Answer from the drawing. Dimensions are ordinates in mm from the lowest x, y and z of the part. A direction names the side the tool comes from. Round coordinates to 2 decimals unless told otherwise and drop trailing zeros. Write each loop counter-clockwise with the first axis right and the second up, starting at its lowest first coordinate (ties: lowest second). Pieces come first, ordered by that corner, then holes. Notation, with made-up numbers: (12, 61) -> (59, 61) arc R26 cw to (59, 75) -> close; hole circle Ø4 at (-14, -28). An arc over 180 degrees is marked (long way). Return JSON: item names as keys, results as strings. Group by question number.
(1) A cutting plane is placed at C-C on z = 441.5. Give the vertices of the cut face in (x, y), then the cut area to 3 significant figures.
(2) Straight lines are drawn through the part: line 1 (Z direction, x = 84, y = 431.5); line 2 (Y direction, x = 386.5, z = 394); line 3 (X direction, y = 801, z = 392). For each, find the intervals that lie inside material, in ascending order.
(3) The mould has two halves that part along Z. Classify the marked faces 3 and 4: released by +Z, released by -Z, zero draft, split by the parting line, or undercut.
(4) A cutting plane is placed at A-A on y = 391.5. Give the vertices of the cut face in (x, z), then the cut area to 3 significant figures.
(5) A cutting plane is placed at D-D on y = 646. Give the vertices of the cut face in (x, z), then the cut area to 3 significant figures.
(6) For the marked faces 1 and 2, determine the directions among +Z, -Z, +X, -X, +Y, -Y from which every point of the face is accessible in a straight line to the end or side of a thin tool.
(7) A cutting plane is placed at B-B on x = 486. Give the vertices of the cut face in (y, z).
(8) Given pin 1 (10 mm diameter, centred on y = 753, z = 78.5, fed in from -X); pin 2 (21 mm diameter, centred on y = 274, z = 9, fed in from +X); pin 3 (12 mm diameter, centred on x = 269, z = 115.5, fed in from +Y), each flat-ended and moving along its own axis, determine where each tip first touches the part or whether it passes through.
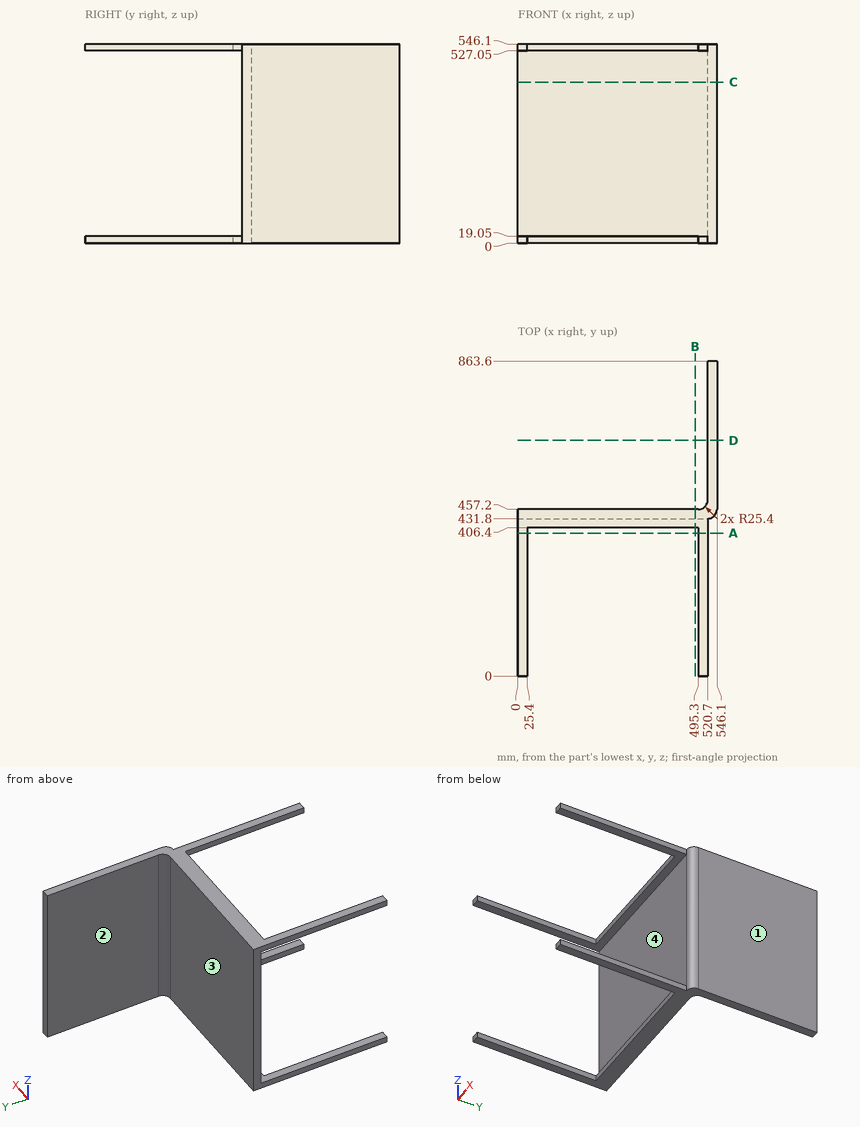
Checks:
{
 "1": {"outline": "(0, 431.8) -> (520.7, 431.8) arc R25.4 ccw to (546.1, 457.2) -> (546.1, 863.6) -> (520.7, 863.6) -> (520.7, 482.6) arc R25.4 cw to (495.3, 457.2) -> (0, 457.2) -> close", "area": "24,200 mm^2"},
 "2": {"line 1": "z = 0 to 19.05, 527.05 to 546.1", "line 2": "y = 431.8 to 457.2", "line 3": "x = 520.7 to 546.1"},
 "3": {"face 3": "zero draft", "face 4": "undercut"},
 "4": {"outline": "(0, 0) -> (25.4, 0) -> (25.4, 19.05) -> (0, 19.05) -> close; (0, 527.05) -> (25.4, 527.05) -> (25.4, 546.1) -> (0, 546.1) -> close; (495.3, 0) -> (520.7, 0) -> (520.7, 19.05) -> (495.3, 19.05) -> close; (495.3, 527.05) -> (520.7, 527.05) -> (520.7, 546.1) -> (495.3, 546.1) -> close", "area": "1,940 mm^2"},
 "5": {"outline": "(520.7, 0) -> (546.1, 0) -> (546.1, 546.1) -> (520.7, 546.1) -> close", "area": "13,900 mm^2"},
 "6": {"face 1": "+Z, -Z, +X, +Y, -Y", "face 2": "+Z, -Z, -X, +Y"},
 "7": {"outline": "(406.4, 0) -> (457.2, 0) -> (457.2, 546.1) -> (406.4, 546.1) -> (406.4, 527.05) -> (431.8, 527.05) -> (431.8, 19.05) -> (406.4, 19.05) -> close"},
 "8": {"pin 1": "stops at x = 520.7", "pin 2": "stops at x = 520.7", "pin 3": "stops at y = 457.2"}
}
